Source: CAD feature listing. Evaluate the final solid. Frame: model axes, mm. A direction names the side the tool comes from. Round coordinates to 2 decimals unless told otherwise and drop trailing zeros. Use one line per item in the form item = value. Start each with the question number.
Q1. Material intervals for probe 1 along X at (y, z) = (49.5, 220); probe 2 along X at (y, z) = (111.5, 221); probe 3 along Z at (x, y) = (-230, 127), sorted ascending.
Q2. Contact query for a flat-ended pin moving along its axis: pin 1 (2 mm diameter, centred on y = 37, z = 196.5, fed in from -X). Output: stop coordinate, or through.
Q3. Reachability of faces 1 (the flat face through (235, 114, 148)), 2 (the flat face through (235, 33, 160)), 3 (the flat face through (-3, 113, 15)), 4 (the flat face through (-235, 58.481, 74)) from +Z, -Z, +X, -X, +Y, -Y: full face, straight path, thin tool, end or side. Return the list, or none.
from build123d import *

# Parameters (mm, degrees)
BOSS_EXTRUDE1_DEPTH = 300
SKETCH2_W           = 15
SKETCH2_H           = 10
CUT_EXTRUDE1_DEPTH  = 603.07972894
SKETCH4_W           = 130
SKETCH4_H           = 10
CUT_EXTRUDE2_DEPTH  = 30
SKETCH7_W           = 130
SKETCH7_H           = 10
CUT_EXTRUDE3_DEPTH  = 30
CHAMFER1_SIZE       = 10
CHAMFER2_SIZE       = 10
CHAMFER3_SIZE       = 10


with BuildPart() as part:
    # Sketch1 → Boss-Extrude1 (new body)
    with BuildSketch(Plane.XY):
        Polygon((250, 118.480565371), (235, 118.480565371), (235, 108.480565371), (250, 108.480565371), (250, -150), (-250, -150), (-250, 108.480565371), (-235, 108.480565371), (-235, 118.480565371), (-250, 118.480565371), (-250, 150), (250, 150), align=None)
    extrude(amount=BOSS_EXTRUDE1_DEPTH)

    # Sketch2 → Cut-Extrude1 (cut, through all)
    with BuildSketch(Plane.ZY.offset(250)):
        with Locations((292.5, 113.480565371)):
            Rectangle(SKETCH2_W, SKETCH2_H)
        with Locations((7.5, 113.480565371)):
            Rectangle(SKETCH2_W, SKETCH2_H)
    extrude(amount=-CUT_EXTRUDE1_DEPTH, mode=Mode.SUBTRACT)

    # Sketch4 → Cut-Extrude2 (cut)
    with BuildSketch(Plane.ZY.offset(250)):
        with Locations((75, 93.480565371)):
            Rectangle(SKETCH4_W, SKETCH4_H)
        with Locations((225, 93.480565371)):
            Rectangle(SKETCH4_W, SKETCH4_H)
        with Locations((225, 73.480565371)):
            Rectangle(SKETCH4_W, SKETCH4_H)
        with Locations((225, 53.480565371)):
            Rectangle(SKETCH4_W, SKETCH4_H)
        with Locations((225, 33.480565371)):
            Rectangle(SKETCH4_W, SKETCH4_H)
        with Locations((225, 13.480565371)):
            Rectangle(SKETCH4_W, SKETCH4_H)
        with Locations((225, -6.519434629)):
            Rectangle(SKETCH4_W, SKETCH4_H)
        with Locations((75, 73.480565371)):
            Rectangle(SKETCH4_W, SKETCH4_H)
        with Locations((75, 53.480565371)):
            Rectangle(SKETCH4_W, SKETCH4_H)
        with Locations((75, 33.480565371)):
            Rectangle(SKETCH4_W, SKETCH4_H)
        with Locations((75, 13.480565371)):
            Rectangle(SKETCH4_W, SKETCH4_H)
        with Locations((75, -6.519434629)):
            Rectangle(SKETCH4_W, SKETCH4_H)
    extrude(amount=-CUT_EXTRUDE2_DEPTH, mode=Mode.SUBTRACT)

    # Sketch7 → Cut-Extrude3 (cut)
    with BuildSketch(Plane(origin=(250, 0, 0), x_dir=(0, 0, -1), z_dir=(1, 0, 0))):
        with Locations((-225, 93.480565371)):
            Rectangle(SKETCH7_W, SKETCH7_H)
        with Locations((-75, 93.480565371)):
            Rectangle(SKETCH7_W, SKETCH7_H)
        with Locations((-75, 73.480565371)):
            Rectangle(SKETCH7_W, SKETCH7_H)
        with Locations((-75, 53.480565371)):
            Rectangle(SKETCH7_W, SKETCH7_H)
        with Locations((-75, 33.480565371)):
            Rectangle(SKETCH7_W, SKETCH7_H)
        with Locations((-75, 13.480565371)):
            Rectangle(SKETCH7_W, SKETCH7_H)
        with Locations((-75, -6.519434629)):
            Rectangle(SKETCH7_W, SKETCH7_H)
        with Locations((-225, 73.480565371)):
            Rectangle(SKETCH7_W, SKETCH7_H)
        with Locations((-225, 53.480565371)):
            Rectangle(SKETCH7_W, SKETCH7_H)
        with Locations((-225, 33.480565371)):
            Rectangle(SKETCH7_W, SKETCH7_H)
        with Locations((-225, 13.480565371)):
            Rectangle(SKETCH7_W, SKETCH7_H)
        with Locations((-225, -6.519434629)):
            Rectangle(SKETCH7_W, SKETCH7_H)
    extrude(amount=-CUT_EXTRUDE3_DEPTH, mode=Mode.SUBTRACT)

    # Chamfer1
    chamfer1_edges = [part.edges().sort_by_distance(p)[0] for p in [
        (0, 150, 0),
        (-250, 150, 150),
        (250, 150, 150),
        (0, 150, 300),
    ]]
    chamfer(chamfer1_edges, length=CHAMFER1_SIZE)

    # Chamfer2
    chamfer2_edges = [part.edges().sort_by_distance(p)[0] for p in [
        (0, 118.480565371, 0),
        (-250, 118.480565371, 150),
        (250, 118.480565371, 150),
        (0, 118.480565371, 300),
    ]]
    chamfer(chamfer2_edges, length=CHAMFER2_SIZE)

    # Chamfer3
    chamfer3_edges = [part.edges().sort_by_distance(p)[0] for p in [
        (250, -20.759717314, 300),
        (250, -20.759717314, 0),
        (-250, -20.759717314, 0),
        (-250, -20.759717314, 300),
    ]]
    chamfer(chamfer3_edges, length=CHAMFER3_SIZE - 0.0001)  # a hair under: the kernel refuses the full size


solid = part.part
Results list:
q1.probe_1 = -220 to 220
q1.probe_2 = -235 to 235
q1.probe_3 = 1.48 to 298.52
q2.pin_1 = -220
q3.face_1 = +Z, -Z, +X
q3.face_2 = +X
q3.face_3 = -Z, +X, -X
q3.face_4 = -X
